from build123d import *

# Parameters (mm, degrees)
F2_R      = 15
F3_DEPTH  = 12
F4_R      = 14
F5_DEPTH  = 3
F6_R      = 1
F8_DEPTH  = 6
F9_R      = 15
F10_DEPTH = 6
F11_R     = 17.75
F12_DEPTH = 15
F13_R     = 2


with BuildPart() as f1:
    # F0 (on Front) → F1 (revolve)
    with BuildSketch(Plane.XZ):
        with BuildLine():
            Line((15, 39.5324291697), (0, 39.5324291697))
            Line((0, 39.5324291697), (0, -68.4675708303))
            Line((0, -68.4675708303), (15, -68.4675708303))
            Line((15, -68.4675708303), (20, -60.9842560568))
            ThreePointArc((20, -60.9842560568), (37.9128784748, -50.7687738723), (45, -31.4038571413))
            Line((45, -31.4038571413), (45, -11.4038571413))
            ThreePointArc((45, -11.4038571413), (37.4032174761, 13.3287561425), (17.2325892015, 29.5324291697))
            Line((17.2325892015, 29.5324291697), (15, 39.5324291697))
        make_face()
    revolve(axis=Axis((0, 0, -14.4675708303), (0, 0, -1)))

    # F2 (on face) → F3 (join)
    with BuildSketch(Plane.XY.offset(39.5324291697)):
        Polygon((9.237604307, -16), (18.4752086141, 0), (9.237604307, 16), (-9.237604307, 16), (-18.4752086141, 0), (-9.237604307, -16), align=None)
        Circle(F2_R, mode=Mode.SUBTRACT)
        Polygon((9.237604307, -16), (18.4752086141, 0), (9.237604307, 16), (-9.237604307, 16), (-18.4752086141, 0), (-9.237604307, -16), align=None)
    extrude(amount=F3_DEPTH)

    # F4 (on face) → F5 (join)
    with BuildSketch(Plane.XY.offset(51.5324291697)):
        Circle(F4_R)
    extrude(amount=F5_DEPTH)

    # F6
    f6_edges = [f1.edges().sort_by_distance(p)[0] for p in [
        (-14, 0, 54.532429),
    ]]
    fillet(f6_edges, radius=F6_R)

    # F7 (on face) → F8 (join)
    with BuildSketch(Plane.XY.offset(54.5324291697)):
        Polygon((4.3301270189, -7.5), (8.0829037687, -1), (1, -1), (1, -7.5), align=None)
        Polygon((-1, -7.5), (-1, -1), (-8.0829037687, -1), (-4.3301270189, -7.5), align=None)
        Polygon((1, 1), (8.0829037687, 1), (4.3301270189, 7.5), (1, 7.5), align=None)
        Polygon((-8.0829037687, 1), (-1, 1), (-1, 7.5), (-4.3301270189, 7.5), align=None)
    extrude(amount=F8_DEPTH)

    # F9 (on face) → F10 (join)
    with BuildSketch(Plane(origin=(0, 0, -68.4675708303), x_dir=(1, 0, 0), z_dir=(0, 0, -1))):
        Polygon((10.3923048454, -18), (20.7846096908, 0), (10.3923048454, 18), (-10.3923048454, 18), (-20.7846096908, 0), (-10.3923048454, -18), align=None)
        Circle(F9_R, mode=Mode.SUBTRACT)
        Polygon((10.3923048454, -18), (20.7846096908, 0), (10.3923048454, 18), (-10.3923048454, 18), (-20.7846096908, 0), (-10.3923048454, -18), align=None)
    extrude(amount=F10_DEPTH)

    # F11 (on face) → F12 (join)
    with BuildSketch(Plane(origin=(0, 0, -74.4675708303), x_dir=(1, 0, 0), z_dir=(0, 0, -1))):
        Circle(F11_R)
    extrude(amount=F12_DEPTH)

    # F13
    f13_edges = [f1.edges().sort_by_distance(p)[0] for p in [
        (-17.75, 0, -89.467571),
    ]]
    fillet(f13_edges, radius=F13_R)


solid = f1.part
The listing builds one solid part. Answer for the finished solid, in the listing's coordinates (mm). A direction names the side the tool comes from. Coordinates: 2 decimals unless noted, no trailing zeros. Loops run counter-clockwise (first coordinate to the right, second up) from the corner with the lowest first, then second, coordinate; pieces in that order, holes last. Notation, with made-up numbers: (-23, -33.5) -> (19, -33.5) arc R27 ccw to (19, -12.5) -> close; hole circle Ø2 at (66, -21). An arc over 180 degrees is marked (long way). Write item = value, one per line. Start each with the question number.
1) A cutting plane is placed at A-A (z = 37.5). Give the vertices of the cut face in (x, y).
2) Given pin 1 Ø2 at (x, z) = (9.5, 27.5) entering from -Y; pin 2 Ø5 at (x, z) = (-4, -71) entering from +Y; pin 3 Ø8 at (y, z) = (26.5, 1) entering from -X; pin 4 Ø8 at (x, y) = (17, -9) entering from -Z, each flat-ended and moving along its own axis, determine where each tip first touches the part or whether it passes through.
3) Straight lines are drawn through the part: line 1 (X direction, y = -35, z = -19); line 2 (Z direction, x = 17, y = -36.5); line 3 (X direction, y = 38.5, z = -23). For each, find the intervals that lie inside material, in ascending order. Write a range as from..to.
4) The mould has two halves that part along X. Classify faces 1 (the face through (-1, -4, 57)), 2 (the face through (4, -4, 60.532)), 3 (the face through (-13.92, -7.89, 45.45)): released by +X, released by -X, zero draft, split by the parting line, or undercut.
5) A tool of negligible diameter and unlimited length cuts with its end or side. For faces 4 (the face through (6.18, -4.295, 57.49)), 5 (the face through (-15.661, 8.874, -71.426)), 6 (the face through (-1, 4, 57)), 7 (the face through (-13.8, 8.1, 45.4)), 8 (the face through (0, 18, -71)), from which of +Z, -Z, +X, -X, +Y, -Y can it reach the whole face along a straight path? Write none if from no direction.
Responses:
q1.outline = circle Ø30.91 at (0, 0)
q2.pin_1 = -21.44
q2.pin_2 = 18
q2.pin_3 = -37.21
q2.pin_4 = -89.47
q3.line_1 = -28.28..28.28
q3.line_2 = -47.58..8.47
q3.line_3 = -23.3..23.3
q4.face_1 = undercut
q4.face_2 = zero draft
q4.face_3 = released by -X
q5.face_4 = +Z, +X, -Y
q5.face_5 = -Z, -X, +Y
q5.face_6 = +Z, +Y, -Y
q5.face_7 = +Z, -X, +Y
q5.face_8 = -Z, +X, -X, +Y
